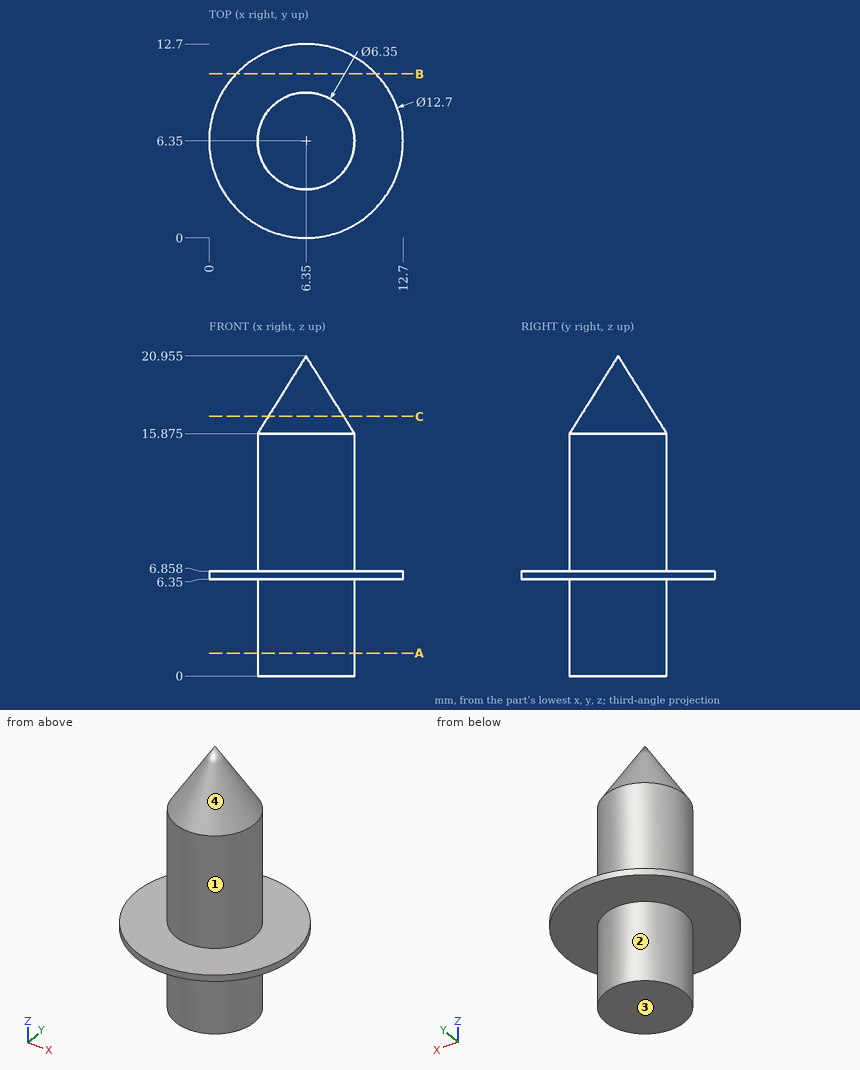
The figure shows three views and two pictorial views of one solid part (mm, origin at its lowest corner). Answer the questions. A direction names the side the tool comes from. Coordinates: 2 decimals unless noted, no trailing zeros. Loops run counter-clockwise (first coordinate to the right, second up) from the corner with the lowest first, then second, coordinate; pieces in that order, holes last. Notation, with made-up numbers: (44.25, 44) - (57.25, 44) arc R23 cw to (57.25, 60) - close; hole circle Ø7 at (-11, 15). An arc over 180 degrees is marked (long way). Use a Markdown table: item, result. Add a question column.
1) The mould has two halves that part along X. Classify the marked faces 3 and 4: released by +X, released by -X, zero draft, split by the parting line, or undercut.
2) For the marked faces 1 and 2, determine the directions among +Z, -Z, +X, -X, +Y, -Y from which every point of the face is accessible in a straight line to the end or side of a thin tool.
3) The part is cut by section A-A, the plane z = 1.5. Give the vertices of the cut face in (x, y) (3 decimals), and give its area (3 significant figures).
4) The part is cut by section C-C, the plane z = 17. Give the vertices of the cut face in (x, y).
5) The part is cut by section B-B, the plane y = 10.75. Give the vertices of the cut face in (x, z).
6) Given pin 1 (2 mm diameter, centred on x = 4, y = 2.5, fed in from -Z); pin 2 (1 mm diameter, centred on x = 8.5, z = 17, fed in from -Y); pin 3 (3 mm diameter, centred on x = 9, z = 17, fed in from -Y), each flat-ended and moving along its own axis, determine where each tip first touches the part or whether it passes through.
7) Find the intervals of material crossed by line 1 (Z direction, x = 12.25, y = 8.5); line 2 (X direction, y = 6.25, z = 7), in increasing order.
Here are the results:
| question | item | result |
|---|---|---|
| 1 | face 3 | zero draft |
| 1 | face 4 | split by the parting line |
| 2 | face 1 | +Z |
| 2 | face 2 | -Z |
| 3 | outline | circle Ø6.35 at (6.35, 6.35) |
| 3 | area | 31.7 mm^2 |
| 4 | outline | circle Ø4.94 at (6.35, 6.35) |
| 5 | outline | (1.77, 6.35) - (10.93, 6.35) - (10.93, 6.86) - (1.77, 6.86) - close |
| 6 | pin 1 | stops at z = 6.35 |
| 6 | pin 2 | stops at y = 4.34 |
| 6 | pin 3 | stops at y = 3.64 |
| 7 | line 1 | z = 6.35 to 6.86 |
| 7 | line 2 | x = 3.18 to 9.52 |
